```python
from build123d import *

# Parameters (mm, degrees)
SKETCH71_W                              = 220.8
SKETCH71_H                              = 150
BASE_FLANGE_DEPTH                       = 1
EDGE_FLANGE_SIDE_STRIP_W                = 5.4732
EDGE_FLANGE_SIDE_STRIP_H                = 1
EDGE_FLANGE_SIDE_STRIP_CUT_DEPTH        = 150
EDGE_FLANGE_SIDE_DEPTH                  = 150
EDGE_FLANGE_SIDE_TOP_STRIP_W            = 5.4732
EDGE_FLANGE_SIDE_TOP_STRIP_H            = 1
EDGE_FLANGE_SIDE_TOP_STRIP_CUT_DEPTH    = 150
EDGE_FLANGE_SIDE_TOP_DEPTH              = 150
EDGE_FLANGE_BOTTOM_DEPTH                = 219.0634
EDGE_FLANGE_BOTTOM_TOP_STRIP_W          = 5.4732
EDGE_FLANGE_BOTTOM_TOP_STRIP_H          = 1
EDGE_FLANGE_BOTTOM_TOP_STRIP_CUT_DEPTH  = 203.8
EDGE_FLANGE_BOTTOM_TOP_RELIEF_W         = 5.9732
EDGE_FLANGE_BOTTOM_TOP_RELIEF_H         = 0.5
EDGE_FLANGE_BOTTOM_TOP_RELIEF_CUT_DEPTH = 1
EDGE_FLANGE_BOTTOM_TOP_DEPTH            = 203.8
EDGE_FLANGE_SIDE_BOTTOM_STRIP_W         = 5.4732
EDGE_FLANGE_SIDE_BOTTOM_STRIP_H         = 1
EDGE_FLANGE_SIDE_BOTTOM_STRIP_CUT_DEPTH = 35.5268
EDGE_FLANGE_SIDE_BOTTOM_DEPTH           = 35.5268


# Sheet-metal steps are written as plain solids
with BuildPart() as part:
    # Sketch71 → Base-Flange (new body)
    with BuildSketch(Plane(origin=(0, -19.5, 0), x_dir=(1, 0, 0), z_dir=(0, 1, 0))):
        with Locations((110.4, -75.7366)):
            Rectangle(SKETCH71_W, SKETCH71_H)
    extrude(amount=BASE_FLANGE_DEPTH)

    # Edge-Flange-Side strip (across the edge) → Edge-Flange-Side strip cut (cut)
    with BuildSketch(Plane(origin=(220.8, -18.5, 150.7366), x_dir=(-1, 0, 0), z_dir=(0, 0, -1))):
        with Locations((-1, -0.5)):
            Rectangle(EDGE_FLANGE_SIDE_STRIP_W, EDGE_FLANGE_SIDE_STRIP_H)
    extrude(amount=EDGE_FLANGE_SIDE_STRIP_CUT_DEPTH, mode=Mode.SUBTRACT)

    # Edge-Flange-Side section (across the edge) → Edge-Flange-Side (add)
    with BuildSketch(Plane(origin=(220.8, -18.5, 150.7366), x_dir=(-1, 0, 0), z_dir=(0, 0, -1))):
        with BuildLine():
            Line((0, 0.7366), (0, 38))
            Line((0, 38), (1, 38))
            Line((1, 38), (1, 0.7366))
            ThreePointArc((1, 0.7366), (1.215745145, 0.215745145), (1.7366, 0))
            Line((1.7366, 0), (1.7366, -1))
            ThreePointArc((1.7366, -1), (0.508638364, -0.491361636), (0, 0.7366))
        make_face()
    extrude(amount=EDGE_FLANGE_SIDE_DEPTH)

    # Edge-Flange-Side-Top strip (across the edge) → Edge-Flange-Side-Top strip cut (cut)
    with BuildSketch(Plane(origin=(219.8, 19.5, 150.7366), x_dir=(0, -1, 0), z_dir=(0, 0, -1))):
        with Locations((-1, -0.5)):
            Rectangle(EDGE_FLANGE_SIDE_TOP_STRIP_W, EDGE_FLANGE_SIDE_TOP_STRIP_H)
    extrude(amount=EDGE_FLANGE_SIDE_TOP_STRIP_CUT_DEPTH, mode=Mode.SUBTRACT)

    # Edge-Flange-Side-Top section (across the edge) → Edge-Flange-Side-Top (add)
    with BuildSketch(Plane(origin=(219.8, 19.5, 150.7366), x_dir=(0, -1, 0), z_dir=(0, 0, -1))):
        with BuildLine():
            Line((0, 0.7366), (0, 15))
            Line((0, 15), (1, 15))
            Line((1, 15), (1, 0.7366))
            ThreePointArc((1, 0.7366), (1.215745145, 0.215745145), (1.7366, 0))
            Line((1.7366, 0), (1.7366, -1))
            ThreePointArc((1.7366, -1), (0.508638364, -0.491361636), (0, 0.7366))
        make_face()
    extrude(amount=EDGE_FLANGE_SIDE_TOP_DEPTH)

    # Edge-Flange-Bottom section (across the edge) → Edge-Flange-Bottom (add)
    with BuildSketch(Plane(origin=(0, -18.5, 151.4732), x_dir=(0, 0, -1), z_dir=(1, 0, 0))):
        with BuildLine():
            Line((-1, 0.7366), (-1, 38))
            Line((-1, 38), (0, 38))
            Line((0, 38), (0, 0.7366))
            ThreePointArc((0, 0.7366), (0.215745145, 0.215745145), (0.7366, 0))
            Line((0.7366, 0), (0.7366, -1))
            ThreePointArc((0.7366, -1), (-0.491361636, -0.491361636), (-1, 0.7366))
        make_face()
    extrude(amount=EDGE_FLANGE_BOTTOM_DEPTH)

    # Edge-Flange-Bottom-Top strip (across the edge) → Edge-Flange-Bottom-Top strip cut (cut)
    with BuildSketch(Plane(origin=(0, 19.5, 151.4732), x_dir=(0, -1, 0), z_dir=(1, 0, 0))):
        with Locations((-1, -0.5)):
            Rectangle(EDGE_FLANGE_BOTTOM_TOP_STRIP_W, EDGE_FLANGE_BOTTOM_TOP_STRIP_H)
    extrude(amount=EDGE_FLANGE_BOTTOM_TOP_STRIP_CUT_DEPTH, mode=Mode.SUBTRACT)

    # Edge-Flange-Bottom-Top relief (on the sheet) → Edge-Flange-Bottom-Top relief cut (cut)
    with BuildSketch(Plane(origin=(0, 17.7634, 151.4732), x_dir=(0, -1, 0), z_dir=(0, 0, -1))):
        with Locations((-2.4866, -204.05)):
            Rectangle(EDGE_FLANGE_BOTTOM_TOP_RELIEF_W, EDGE_FLANGE_BOTTOM_TOP_RELIEF_H)
    extrude(amount=-EDGE_FLANGE_BOTTOM_TOP_RELIEF_CUT_DEPTH, mode=Mode.SUBTRACT)

    # Edge-Flange-Bottom-Top section (across the edge) → Edge-Flange-Bottom-Top (add)
    with BuildSketch(Plane(origin=(0, 19.5, 151.4732), x_dir=(0, -1, 0), z_dir=(1, 0, 0))):
        with BuildLine():
            Line((0, 0.7366), (0, 15))
            Line((0, 15), (1, 15))
            Line((1, 15), (1, 0.7366))
            ThreePointArc((1, 0.7366), (1.215745145, 0.215745145), (1.7366, 0))
            Line((1.7366, 0), (1.7366, -1))
            ThreePointArc((1.7366, -1), (0.508638364, -0.491361636), (0, 0.7366))
        make_face()
    extrude(amount=EDGE_FLANGE_BOTTOM_TOP_DEPTH)

    # Edge-Flange-Side-Bottom strip (across the edge) → Edge-Flange-Side-Bottom strip cut (cut)
    with BuildSketch(Plane(origin=(219.8, -17.7634, 150.7366), x_dir=(0, 0, -1), z_dir=(0, 1, 0))):
        with Locations((-1, -0.5)):
            Rectangle(EDGE_FLANGE_SIDE_BOTTOM_STRIP_W, EDGE_FLANGE_SIDE_BOTTOM_STRIP_H)
    extrude(amount=EDGE_FLANGE_SIDE_BOTTOM_STRIP_CUT_DEPTH, mode=Mode.SUBTRACT)

    # Edge-Flange-Side-Bottom section (across the edge) → Edge-Flange-Side-Bottom (add)
    with BuildSketch(Plane(origin=(219.8, -17.7634, 150.7366), x_dir=(0, 0, -1), z_dir=(0, 1, 0))):
        with BuildLine():
            Line((0, 0.7366), (0, 7.5))
            Line((0, 7.5), (1, 7.5))
            Line((1, 7.5), (1, 0.7366))
            ThreePointArc((1, 0.7366), (1.215745145, 0.215745145), (1.7366, 0))
            Line((1.7366, 0), (1.7366, -1))
            ThreePointArc((1.7366, -1), (0.508638364, -0.491361636), (0, 0.7366))
        make_face()
    extrude(amount=EDGE_FLANGE_SIDE_BOTTOM_DEPTH)

    # Mirror-Vertical: part across plane


with BuildPart() as part_1:
    add(part.part)
    add(part.part.mirror(Plane(origin=(0, -18.5, 0.7366), x_dir=(0, 0, 1), z_dir=(1, 0, 0))))


solid = part_1.part
```
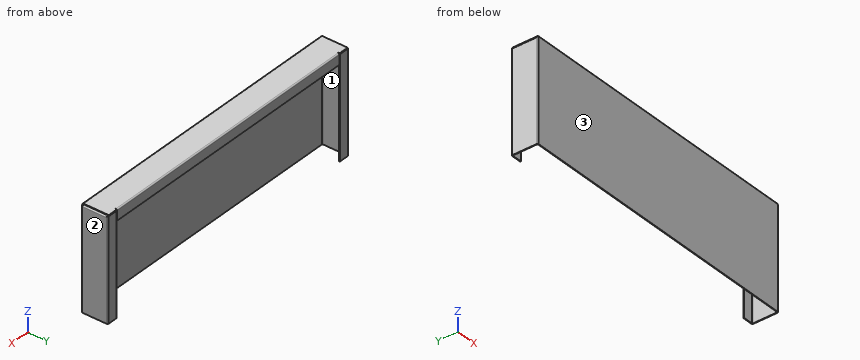
For this review, take the finished solid that the model builds, in its own axes (mm). Face numbers are marked on the shaded views. Coordinates: 2 decimals unless noted, no trailing zeros. Write each loop counter-clockwise with the first axis right and the second up, starting at its lowest first coordinate (ties: lowest second). Pieces come first, ordered by that corner, then holes.
(1) For pin 1 Ø10 at (x, z) = (5, 116) entering from +Y; pin 2 Ø0.8 at (y, z) = (8.5, 150.5) entering from -X; pin 3 Ø0.8 at (x, z) = (220.5, 150) entering from +Y, all flat-tipped, find the tip position at first contact; note any pin that passes through.
(2) The part is to be moulded in two halves that separate along Y. For the marked faces 1, 2 and 3, say which applies: +Y half, -Y half, draft (parallel to the pull), parting line (faces both ways), or undercut.
(3) Add section A-A on y = 2. Give the boundary of the cut face in (x, z).
(4) Wall thickness on probe 1 along X at (y, z) = (-15.5, 36); probe 2 along Y at (x, z) = (-169.5, 142); probe 3 along Z at (x, y) = (-144.5, 7.5): over which ranges is each line inside the solid? List them lowest first.
(5) Add section B-B on x = -99. Give the boundary of the cut face in (y, z), then the cut area to 3 significant figures.
(6) Add section C-C on z = 31. Give the boundary of the cut face in (x, y), then the cut area to 3 significant figures.
Answer sheet:
1. pin 1: stops at y = -18.5
1. pin 2: stops at x = -220.41
1. pin 3: stops at y = 19.16
2. face 1: undercut
2. face 2: draft
2. face 3: -Y half
3. outline: (-220.8, 0.74) - (-219.8, 0.74) - (-219.8, 149) arc R0.74 cw to (-219.06, 149.74) - (-212.3, 149.74) - (-212.3, 150.74) - (-219.06, 150.74) arc R1.74 ccw to (-220.8, 149) - close; (-219.06, 151.47) - (219.06, 151.47) - (219.06, 152.47) - (-219.06, 152.47) - close; (212.3, 149.74) - (219.06, 149.74) arc R0.74 cw to (219.8, 149) - (219.8, 0.74) - (220.8, 0.74) - (220.8, 149) arc R1.74 ccw to (219.06, 150.74) - (212.3, 150.74) - close
4. probe 1: x = -220.8 to -219.8, 219.8 to 220.8
4. probe 2: y = -19.5 to -18.5, 18.5 to 19.5
4. probe 3: z = 151.47 to 152.47
5. outline: (-19.5, 0.74) - (-18.5, 0.74) - (-18.5, 150.74) arc R0.74 cw to (-17.76, 151.47) - (17.76, 151.47) arc R0.74 cw to (18.5, 150.74) - (18.5, 136.47) - (19.5, 136.47) - (19.5, 150.74) arc R1.74 ccw to (17.76, 152.47) - (-17.76, 152.47) arc R1.74 ccw to (-19.5, 150.74) - close
5. area: 204 mm2
6. outline: (-220.8, -17.76) arc R1.74 ccw to (-219.06, -19.5) - (219.06, -19.5) arc R1.74 ccw to (220.8, -17.76) - (220.8, 17.76) arc R1.74 ccw to (219.06, 19.5) - (204.8, 19.5) - (204.8, 18.5) - (219.06, 18.5) arc R0.74 cw to (219.8, 17.76) - (219.8, -17.76) arc R0.74 cw to (219.06, -18.5) - (-219.06, -18.5) arc R0.74 cw to (-219.8, -17.76) - (-219.8, 17.76) arc R0.74 cw to (-219.06, 18.5) - (-204.8, 18.5) - (-204.8, 19.5) - (-219.06, 19.5) arc R1.74 ccw to (-220.8, 17.76) - close
6. area: 545 mm2
